The listing builds one solid part. Answer for the finished solid, in the listing's coordinates (mm). A direction names the side the tool comes from. Round coordinates to 2 decimals unless told otherwise and drop trailing zeros. Loops run counter-clockwise (first coordinate to the right, second up) from the corner with the lowest first, then second, coordinate; pieces in that order, holes last. Notation, with made-up numbers: (-15, -13.5) - (2, -13.5) arc R22 ccw to (2, 19.5) - close; hole circle Ø8 at (-19, -17.75). An arc over 180 degrees is marked (long way). Write item = value, one per line. Start each with the question number.
1) Section A-A, the plane z = 95.5 is taken. Determine the outline of the cut face in (x, y).
2) Straight lines are drawn through the part: line 1 along X through (y, z) = (-2.5, 82); line 2 along X through (y, z) = (33, 86); line 3 along Z through (x, y) = (-0.5, -25). For each, find the intervals that lie inside material, in ascending order.
3) For a pull along X with two mould halves and no side action, classify faces 1 (the cylindrical face through (-65.979, 31.445, 5.505)), 2 (the cylindrical face through (1.65, 0.56, -149.98)), 3 (the flat face through (-45, -1, 109)), 4 (the flat face through (60, 0, 150)) as released by +X, released by -X, zero draft, split by the parting line, or undercut.
4) A tool of negligible diameter and unlimited length cuts with its end or side. For faces 5 (the flat face through (1, -1, 70)), 6 (the cylindrical face through (-56.46, -26.94, 144.76)), from which of +Z, -Z, +X, -X, +Y, -Y can it reach the whole face along a straight path? Write none if from no direction.
5) Given pin 1 Ø1 at (x, y) = (59.5, 8.5) entering from -Z; pin 2 Ø2 at (x, y) = (2, -26.5) entering from -Z; pin 3 Ø10 at (x, y) = (-33.5, -1.5) entering from -Z, each flat-ended and moving along its own axis, determine where each tip first touches the part or whether it passes through.
6) Section B-B, the plane y = 2 is taken. Determine the outline of the cut face in (x, z).
7) Section C-C, the plane z = -39.5 is taken. Determine the outline of the cut face in (x, y), and give its area (3 significant figures).
8) Section D-D, the plane z = 129 is taken. Determine the outline of the cut face in (x, y), and give its area (3 significant figures).
from build123d import *

# Parameters (mm, degrees)
BOSS_EXTRUDE1_DEPTH      = 150
BOSS_EXTRUDE1_DEPTH_BACK = 150
SKETCH2_OUTSIDE_W        = 370.964
SKETCH2_OUTSIDE_H        = 150.964
CUT_EXTRUDE1_DEPTH       = 150
CUT_EXTRUDE2_REACH       = 187.809
SKETCH6_OUTSIDE_W        = 220.96400000000003
SKETCH6_OUTSIDE_H        = 370.964
CUT_EXTRUDE3_DEPTH       = 186.8090417606205


with BuildPart() as part:
    # Sketch1 → Boss-Extrude1 (new, two sides: drawn at the far end of the back side and taken through both)
    with BuildSketch(Plane.XY.offset(-BOSS_EXTRUDE1_DEPTH_BACK)):
        with BuildLine():
            Line((-44.999999999999986, -39.99999999999999), (45.000000000000014, -39.99999999999999))
            ThreePointArc((45.000000000000014, -39.99999999999999), (66.21320343559644, -31.21320343559642), (75.00000000000001, -10.000000000000002))
            Line((75.00000000000001, -10.000000000000002), (75.00000000000001, 10.000000000000002))
            ThreePointArc((75.00000000000001, 10.000000000000002), (66.21320343559645, 31.213203435596434), (45.000000000000014, 40.00000000000001))
            Line((45.000000000000014, 40.00000000000001), (-44.999999999999986, 40.00000000000001))
            ThreePointArc((-44.999999999999986, 40.00000000000001), (-66.21320343559641, 31.213203435596427), (-74.99999999999999, 10.000000000000002))
            Line((-74.99999999999999, 10.000000000000002), (-74.99999999999999, -10.000000000000002))
            ThreePointArc((-74.99999999999999, -10.000000000000002), (-66.2132034355964, -31.213203435596427), (-44.999999999999986, -39.99999999999999))
        make_face()
    extrude(amount=BOSS_EXTRUDE1_DEPTH + BOSS_EXTRUDE1_DEPTH_BACK)

    # Sketch2 outside → Cut-Extrude1 (cut)
    with BuildSketch(Plane(origin=(75.00000000000001, 0, 0), x_dir=(0, 0, -1), z_dir=(1, 0, 0))):
        Rectangle(SKETCH2_OUTSIDE_W, SKETCH2_OUTSIDE_H)
        with BuildLine():
            Line((150, 40.00000000000001), (-120, 39.999999999999986))
            ThreePointArc((-120, 39.999999999999986), (-141.21320343559643, 31.21320343559642), (-150, 9.999999999999991))
            Line((-150, 9.999999999999991), (-150, -9.999999999999991))
            ThreePointArc((-150, -9.999999999999991), (-141.21320343559643, -31.213203435596412), (-120, -39.999999999999986))
            Line((-120, -39.999999999999986), (150, -39.999999999999964))
            Line((150, -39.999999999999964), (150, 40.00000000000001))
        make_face(mode=Mode.SUBTRACT)
    extrude(amount=-CUT_EXTRUDE1_DEPTH, mode=Mode.SUBTRACT)

    # Sketch3 → Cut-Extrude2 (cut, up to next)
    with BuildSketch(Plane.XZ.offset(39.99999999999999), mode=Mode.PRIVATE) as cut_extrude2_sk1:
        Polygon((-44.99999999999978, 150), (45, 150), (45.000000000000014, 69.99999999999999), (-44.99999999999977, 69.99999999999999), align=None)
    cut_extrude2_tool1 = extrude(cut_extrude2_sk1.sketch, amount=-CUT_EXTRUDE2_REACH, mode=Mode.PRIVATE) & part.part
    add(cut_extrude2_tool1.solids().sort_by_distance((0, -40, 110))[0], mode=Mode.SUBTRACT)

    # Sketch6 outside → Cut-Extrude3 (cut, through all)
    with BuildSketch(Plane(origin=(0, 40.00000000000001, 0), x_dir=(1, 0, 0), z_dir=(0, 1, 0))):
        Rectangle(SKETCH6_OUTSIDE_W, SKETCH6_OUTSIDE_H)
        with BuildLine():
            Line((-75, 75), (-74.99999999999999, 0))
            Line((-74.99999999999999, 0), (-74.99999999999999, -150))
            Line((-74.99999999999999, -150), (75.00000000000001, -150))
            Line((75.00000000000001, -150), (75.00000000000001, 0))
            Line((75.00000000000001, 0), (75, 75))
            ThreePointArc((75, 75), (-9.29e-15, 149.99999999999997), (-75, 75))
        make_face(mode=Mode.SUBTRACT)
    extrude(amount=-CUT_EXTRUDE3_DEPTH, mode=Mode.SUBTRACT)


solid = part.part
Geometry check:
q1.outline = (-75, -10) arc R30 ccw to (-45, -40) - (-45, 40) arc R30 ccw to (-75, 10) - close; (45, -40) arc R30 ccw to (75, -10) - (75, 10) arc R30 ccw to (45, 40) - close
q2.line_1 = -75 to -45, 45 to 75
q2.line_2 = -64.26 to -45, 45 to 64.26
q2.line_3 = -150 to 70
q3.face_1 = released by -X
q3.face_2 = split by the parting line
q3.face_3 = undercut
q3.face_4 = zero draft
q4.face_5 = +Z, +Y, -Y
q4.face_6 = +Z, +X, -X, -Y
q5.pin_1 = -121.3
q5.pin_2 = -149.99
q5.pin_3 = -144.37
q6.outline = (-75, -75) arc R75 ccw to (75, -75) - (75, 150) - (45, 150) - (45, 70) - (-45, 70) - (-45, 150) - (-75, 150) - close
q7.outline = (-75, -10) arc R30 ccw to (-45, -40) - (45, -40) arc R30 ccw to (75, -10) - (75, 10) arc R30 ccw to (45, 40) - (-45, 40) arc R30 ccw to (-75, 10) - close
q7.area = 11,200 mm2
q8.outline = (-75, -10) arc R30 ccw to (-54, -38.62) - (-45, -38.62) - (-45, 38.62) - (-54, 38.62) arc R30 ccw to (-75, 10) - close; (45, -38.62) - (54, -38.62) arc R30 ccw to (75, -10) - (75, 10) arc R30 ccw to (54, 38.62) - (45, 38.62) - close
q8.area = 3,990 mm2
